Work out the finished part from the listing and answer in its coordinate system (mm). Coordinates: 2 decimals unless noted, no trailing zeros. Order: outer loops, then holes, each group sorted by start corner. A loop starts at its lowest first (then second) coordinate and runs counter-clockwise, first axis right, second up. Notation, with made-up numbers: (66.25, 71.25) -> (90.25, 71.25) arc R8 ccw to (90.25, 81.25) -> close; hole circle Ø10 at (5, 36.5). An arc over 180 degrees is marked (long way). Write item = value, one per line. Start each with the question number.
Q1. Straight lines are drawn through the part: L1, parallel to Z at x = 163, y = -1.6; L2, parallel to Z at x = 19, y = -0.9; L3, parallel to Z at x = 307, y = -1.6. For each, find the intervals that lie inside material, in ascending order. Write a range as from..to.
Q2. The part is cut by section C-C, the plane z = 156. Determine the outline of the cut face in (x, y), plus the area to 3 significant figures.
Q3. The part is cut by section B-B, the plane y = -1.2. Count the separate pieces of the cut face and the enclosed holes in it, plus the area to 3 significant figures.
Q4. Flat-ended cylindrical pins translate along their axes: pin 1 (1.5 mm diameter, centred on x = 350.5, y = -2, fed in from +Z); pin 2 (1.5 mm diameter, centred on y = -1, z = 199, fed in from +X). Find the tip coordinate at first contact, or state that the pin passes through.
Q5. The part is cut by section D-D, the plane x = 133. Determine the outline of the cut face in (y, z), plus the area to 3 significant figures.
Q6. The part is cut by section A-A, the plane z = 126. Determine the outline of the cut face in (x, y).
```python
from build123d import *

# Parameters (mm, degrees)
F0_R     = 3
F0_R_2   = 12.5
F1_DEPTH = 3
F2_R     = 5
F3_R     = 5


with BuildPart() as f1:
    # F0 (on Front) → F1 (new body)
    with BuildSketch(Plane.XZ):
        Polygon((0, 252), (0, 0), (405, 0), (405, 168), (326, 168), (326, 252), align=None)
        with Locations((19, 19)):
            Circle(F0_R, mode=Mode.SUBTRACT)
        with Locations((163, 96)):
            Circle(F0_R_2, mode=Mode.SUBTRACT)
        with Locations((386, 19)):
            Circle(F0_R, mode=Mode.SUBTRACT)
        with Locations((133, 126)):
            Circle(F0_R_2, mode=Mode.SUBTRACT)
        with Locations((163, 126)):
            Circle(F0_R_2, mode=Mode.SUBTRACT)
        with Locations((193, 126)):
            Circle(F0_R_2, mode=Mode.SUBTRACT)
        with Locations((163, 156)):
            Circle(F0_R_2, mode=Mode.SUBTRACT)
        with Locations((19, 233)):
            Circle(F0_R, mode=Mode.SUBTRACT)
        with Locations((386, 149)):
            Circle(F0_R, mode=Mode.SUBTRACT)
        with Locations((307, 233)):
            Circle(F0_R, mode=Mode.SUBTRACT)
    extrude(amount=F1_DEPTH)

    # F2
    f2_edges = [f1.edges().sort_by_distance(p)[0] for p in [
        (326, -1.5, 252),
        (405, -1.5, 168),
        (405, -1.5, 0),
        (0, -1.5, 0),
        (0, -1.5, 252),
    ]]
    fillet(f2_edges, radius=F2_R)

    # F3
    f3_edges = [f1.edges().sort_by_distance(p)[0] for p in [
        (326, -1.5, 168),
    ]]
    fillet(f3_edges, radius=F3_R)


solid = f1.part
```
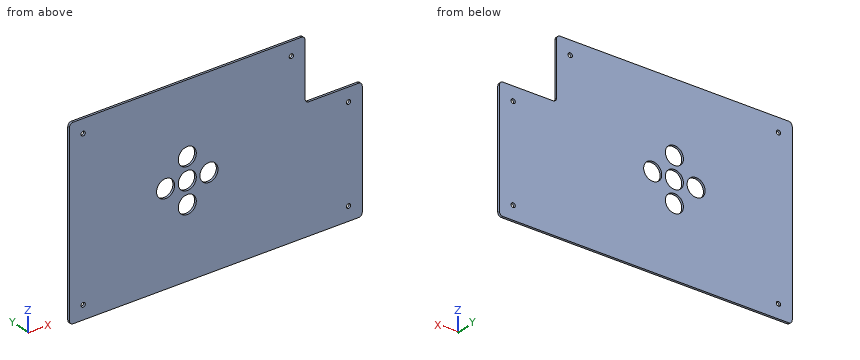
Model answer:
q1.L1 = 0..83.5, 108.5..113.5, 138.5..143.5, 168.5..252
q1.L2 = 0..16, 22..230, 236..252
q1.L3 = 0..230, 236..252
q2.outline = (0, -3) -> (150.5, -3) -> (150.5, 0) -> (0, 0) -> close; (175.5, -3) -> (405, -3) -> (405, 0) -> (175.5, 0) -> close
q2.area = 1,140 mm2
q3.separate_pieces = 1
q3.enclosed_holes = 10
q3.area = 92,800 mm2
q4.pin_1 = 168
q4.pin_2 = 326
q5.outline = (-3, 0) -> (0, 0) -> (0, 113.5) -> (-3, 113.5) -> close; (-3, 138.5) -> (0, 138.5) -> (0, 252) -> (-3, 252) -> close
q5.area = 681 mm2
q6.outline = (0, -3) -> (120.5, -3) -> (120.5, 0) -> (0, 0) -> close; (145.5, -3) -> (150.5, -3) -> (150.5, 0) -> (145.5, 0) -> close; (175.5, -3) -> (180.5, -3) -> (180.5, 0) -> (175.5, 0) -> close; (205.5, -3) -> (405, -3) -> (405, 0) -> (205.5, 0) -> close
